The model under review builds one solid part; all positions refer to its coordinate system, in mm. A direction names the side the tool comes from. Give positions to 0.01 mm unless a question says otherwise; leave off trailing zeros. Write each loop counter-clockwise with the first axis right and the second up, starting at its lowest first coordinate (ties: lowest second). Pieces come first, ordered by that corner, then holes. Notation, with made-up numbers: (76, 83) - (103, 83) arc R12 cw to (103, 100) - close; hole circle Ø11 at (-14, 41). An arc over 180 degrees is marked (long way). Write item = value, one per line.
```python
from build123d import *

# Parameters (mm, degrees)
F0_W     = 72.4
F0_H     = 12.4
F0_W_2   = 69.8
F0_H_2   = 9.8
F0_W_3   = 68.2
F0_H_3   = 8.2
F1_DEPTH = 2
F2_DEPTH = 2.5
F3_R     = 2.5
F4_R     = 2
F5_R     = 1
F6_R     = 1


with BuildPart() as f1:
    # F0 (on Top) → F1 (new body)
    with BuildSketch(Plane.XY):
        with Locations((19.4677342524, 8.0702581361)):
            Rectangle(F0_W, F0_H)
        with Locations((19.4677342524, 8.0702581361)):
            Rectangle(F0_W_2, F0_H_2, mode=Mode.SUBTRACT)
        with Locations((19.4677342524, 8.0702581361)):
            Rectangle(F0_W_2, F0_H_2)
        with Locations((19.4677342524, 8.0702581361)):
            Rectangle(F0_W_3, F0_H_3, mode=Mode.SUBTRACT)
        with Locations((19.4677342524, 8.0702581361)):
            Rectangle(F0_W_3, F0_H_3)
    extrude(amount=-F1_DEPTH)

    # F0 (on Top) → F2 (join)
    with BuildSketch(Plane.XY):
        with Locations((19.4677342524, 8.0702581361)):
            Rectangle(F0_W_2, F0_H_2)
        with Locations((19.4677342524, 8.0702581361)):
            Rectangle(F0_W_3, F0_H_3, mode=Mode.SUBTRACT)
    extrude(amount=F2_DEPTH)

    # F3
    f3_edges = [f1.edges().sort_by_distance(p)[0] for p in [
        (-16.732266, 14.270258, -1),
        (-16.732266, 1.870258, -1),
        (55.667734, 14.270258, -1),
        (55.667734, 1.870258, -1),
    ]]
    fillet(f3_edges, radius=F3_R)

    # F4
    f4_edges = [f1.edges().sort_by_distance(p)[0] for p in [
        (54.367734, 12.970258, 1.25),
        (54.367734, 3.170258, 1.25),
        (-15.432266, 12.970258, 1.25),
        (-15.432266, 3.170258, 1.25),
    ]]
    fillet(f4_edges, radius=F4_R)

    # F5
    f5_edges = [f1.edges().sort_by_distance(p)[0] for p in [
        (53.567734, 3.970258, 1.25),
        (53.567734, 12.170258, 1.25),
        (-14.632266, 3.970258, 1.25),
        (-14.632266, 12.170258, 1.25),
    ]]
    fillet(f5_edges, radius=F5_R)

    # F6
    f6_edges = [f1.edges().sort_by_distance(p)[0] for p in [
        (19.467734, 12.170258, 0),
        (53.567734, 8.070258, 0),
        (19.467734, 3.970258, 0),
        (-14.632266, 8.070258, 0),
    ]]
    fillet(f6_edges, radius=F6_R)


solid = f1.part
```
1. Take a section at B-B on y = 9.5. Give the boundary of the cut face in (x, z).
Findings below:
outline = (-16.73, -2) - (55.67, -2) - (55.67, 0) - (54.37, 0) - (54.37, 2.5) - (53.57, 2.5) - (53.57, 1) arc R1 cw to (52.57, 0) - (-13.63, 0) arc R1 cw to (-14.63, 1) - (-14.63, 2.5) - (-15.43, 2.5) - (-15.43, 0) - (-16.73, 0) - close
2. Take a section at A-A on x = 47.5. Give the boundary of the cut face in (y, z).
Findings below:
outline = (1.87, -2) - (14.27, -2) - (14.27, 0) - (12.97, 0) - (12.97, 2.5) - (12.17, 2.5) - (12.17, 1) arc R1 cw to (11.17, 0) - (4.97, 0) arc R1 cw to (3.97, 1) - (3.97, 2.5) - (3.17, 2.5) - (3.17, 0) - (1.87, 0) - close
3. For line 1 (X direction, y = 9.5, z = 2.2); line 2 (Y direction, x = 10.5, z = 2.25); line 3 (Z direction, x = -8, y = 8.25), list the stretches that pass through material, from the lowest coordinate up. Write a range as from..to.
Findings below:
line_1 = -15.43..-14.63, 53.57..54.37
line_2 = 3.17..3.97, 12.17..12.97
line_3 = -2..0
4. Draft analysis for pull direction Y (two halves, no side actions). For faces 1 (the cylindrical face through (54.916, 13.557, -1.014)), 2 (the flat face through (-14.632, 8, 2)), 3 (the flat face through (-16.732, 8, -1)), state which applies: +Y half, -Y half, draft (parallel to the pull), parting line (faces both ways), or undercut.
Findings below:
face_1 = +Y half
face_2 = undercut
face_3 = draft
5. Insertion check: P1, Ø1.5, axis at x = 45.5, z = 1.5, coming from the -Y side; P2, Ø1.2, axis at x = 17, z = 1, coming from the +Y side; P3, Ø1.9, axis at x = 13.5, y = 7, coming from the +Z side. Each pin has a flat end and moves straight along its axis. Give the tip position at first contact, or say it passes through.
Findings below:
P1 = 3.17
P2 = 12.97
P3 = 0
6. Machinability: for faces 4 (the flat face through (-15.432, 8, 1)), 5 (the flat face through (53.568, 8, 2)), 6 (the cylindrical face through (53.766, 3.741, 1.268)), which of the approach directions +Z, -Z, +X, -X, +Y, -Y give a long, thin tool a straight path to every point of the face, cutting with its end or side? Answer none if there is none.
Findings below:
face_4 = +Z, -X, +Y, -Y
face_5 = +Z
face_6 = +Z, +X, -Y
